Part model, mm, in its own coordinate system. A direction names the side the tool comes from. Give positions to 0.01 mm unless a question says otherwise; leave off trailing zeros. Write each loop counter-clockwise with the first axis right and the second up, starting at its lowest first coordinate (ties: lowest second). Pieces come first, ordered by that corner, then holes. Notation, with made-up numbers: M -8,-21 L 20,-21 A28 ccw 20,15 Z; hole C 25,75.25 d8. An arc over 180 degrees is marked long. Answer as CSV lines item,"result". Start each with the question number.
Item 1: Wall check: L1, parallel to Y at x = -29.55, z = 4.4 (3 decimals); L2, parallel to Y at x = -29.55, z = 0.5 (3 decimals); L3, parallel to X at y = -31.5, z = 2.8. Give the ranges that are in metal, low to high. Write a range as from..to.
Item 2: Band-saw the part on B-B, the plane z = 3.85. Count the separate pieces of the cut face and the enclosed holes in it, then the cut area to 3 significant figures.
Item 3: Band-saw the part on C-C, the plane x = -60. List the corners of the cut face in (y, z), then the cut area to 3 significant figures.
Item 4: Pin check, flat tips, straight feed: pin 1 (5 mm diameter, centred on x = -62.5, y = -35.5, fed in from +Z); pin 2 (4.5 mm diameter, centred on x = -61.3, y = -4.125, fed in from +Z). Stop position of each tip, or through.
Item 5: Two-plate mould, pull along Y, no slides. Class faces 1 (the flat face through (-39, 0, 3)), 2 (the cylindrical face through (-16.3, -8.22, 3.04)), 3 (the flat face through (-65.43, -20, 3)): +Y half, -Y half, draft (parallel to the pull), parting line (faces both ways), or undercut.
Item 6: Band-saw the part on A-A, the plane x = -29.55. List the corners of the cut face in (y, z) (3 decimals), then the cut area to 3 significant figures.
Item 7: 3-axis set-ups, long thin cutter, end or side, ignore diameter. For faces 4 (the flat face through (-59, -36, 1)), 5 (the cylindrical face through (-63.3, -4.04, 0.49)): which of +Z, -Z, +X, -X, +Y, -Y reach the whole face in a straight line?
from build123d import *

# Parameters (mm, degrees)
SKETCH1_W           = 54
SKETCH1_H           = 40
BOSS_EXTRUDE1_DEPTH = 6
SKETCH2_R           = 2
CUT_EXTRUDE2_DEPTH  = 7
SKETCH8_R           = 3
CUT_EXTRUDE6_DEPTH  = 5
SKETCH9_R           = 2.49
CUT_EXTRUDE7_DEPTH  = 6


with BuildPart() as part:
    # Sketch1 → Boss-Extrude1 (new body)
    with BuildSketch(Plane.XY):
        with Locations((-38.43, -20)):
            Rectangle(SKETCH1_W, SKETCH1_H)
    extrude(amount=BOSS_EXTRUDE1_DEPTH)

    # Sketch2 → Cut-Extrude2 (cut, through all)
    with BuildSketch(Plane.XY):
        with Locations((-61.3, -35.875)):
            Circle(SKETCH2_R)
        with Locations((-29.55, -35.875)):
            Circle(SKETCH2_R)
        with Locations((-29.55, -4.125)):
            Circle(SKETCH2_R)
        with Locations((-61.3, -4.125)):
            Circle(SKETCH2_R)
    extrude(amount=CUT_EXTRUDE2_DEPTH, mode=Mode.SUBTRACT)

    # Sketch8 → Cut-Extrude6 (cut)
    with BuildSketch(Plane.XY.offset(6)):
        with Locations((-61.3, -4.125)):
            Circle(SKETCH8_R)
        with Locations((-29.55, -4.125)):
            Circle(SKETCH8_R)
        with Locations((-29.55, -35.875)):
            Circle(SKETCH8_R)
        with Locations((-61.3, -35.875)):
            Circle(SKETCH8_R)
    extrude(amount=-CUT_EXTRUDE6_DEPTH, mode=Mode.SUBTRACT)

    # Sketch9 → Cut-Extrude7 (cut)
    with BuildSketch(Plane.XY.offset(6)):
        with Locations((-44.030806884, -7.27)):
            Circle(SKETCH9_R)
        with Locations((-18.600806884, -7.27)):
            Circle(SKETCH9_R)
        with Locations((-44.030806884, -32.7)):
            Circle(SKETCH9_R)
        with Locations((-18.600806884, -32.7)):
            Circle(SKETCH9_R)
    extrude(amount=-CUT_EXTRUDE7_DEPTH, mode=Mode.SUBTRACT)


solid = part.part
Output:
1,L1,"-40..-38.875, -32.875..-7.125, -1.125..0"
1,L2,"-40..-37.875, -33.875..-6.125, -2.125..0"
1,L3,"-65.43..-46.21, -41.85..-20.78, -16.42..-11.43"
2,separate pieces,"1"
2,enclosed holes,"8"
2,area,"1,970 mm²"
3,outline,"M -40,0 L -37.39,0 L -37.39,1 L -38.58,1 L -38.58,6 L -40,6 Z; M -34.36,0 L -5.64,0 L -5.64,1 L -6.83,1 L -6.83,6 L -33.17,6 L -33.17,1 L -34.36,1 Z; M -2.61,0 L 0,0 L 0,6 L -1.42,6 L -1.42,1 L -2.61,1 Z"
3,area,"180 mm²"
4,pin 1,"z = 6"
4,pin 2,"z = 1"
5,face 1,"+Y half"
5,face 2,"undercut"
5,face 3,"draft"
6,outline,"M -40,0 L -37.875,0 L -37.875,1 L -38.875,1 L -38.875,6 L -40,6 Z; M -33.875,0 L -6.125,0 L -6.125,1 L -7.125,1 L -7.125,6 L -32.875,6 L -32.875,1 L -33.875,1 Z; M -2.125,0 L 0,0 L 0,6 L -1.125,6 L -1.125,1 L -2.125,1 Z"
6,area,"172 mm²"
7,face 4,"+Z"
7,face 5,"+Z, -Z"
